For this review, take the finished solid that the model builds, in its own axes (mm). Face numbers are marked on the shaded views. A direction names the side the tool comes from. Coordinates: 2 decimals unless noted, no trailing zeros. Write each loop counter-clockwise with the first axis right and the second up, starting at its lowest first coordinate (ties: lowest second). Pieces come first, ordered by that corner, then holes. Notation, with made-up numbers: (35, 44.5) - (47, 44.5) arc R27 cw to (47, 69.5) - close; hole circle Ø2 at (31.25, -24.5). An arc over 180 degrees is marked (long way). Use one line per item in the form item = value. Start each with the question number.
1) Mouldability with a two-part tool opening along X and no side actions: class the marked faces 1 and 2 as pulls with the +X half, pulls with the -X half, needs draft (parallel to the pull), parting line crosses it, or undercut.
2) We need section B-B (z = 0). Give the boundary of the cut face in (x, y) (3 decimals), plus the area to 3 significant figures.
3) Insertion check: P1, Ø3.5, axis at x = 43.18, z = 0, coming from the +Y side; P2, Ø1.5, axis at y = 2, z = -2, coming from the +X side; P3, Ø1.5, axis at x = 40.5, y = 0.5, coming from the +Z side; P4, Ø1.6, axis at x = 29.5, y = 2, coming from the -Z side (3 decimals). Each pin has a flat end and moves straight along its axis. Give the tip position at first contact, or say it passes through.
4) We need section C-C (y = 2.7). Give the boundary of the cut face in (x, z) (3 decimals).
5) We need section D-D (x = 31.5). Give the boundary of the cut face in (y, z) (3 decimals).
6) We need section A-A (x = 43.18). Give the boundary of the cut face in (y, z) (3 decimals).
7) For L1, parallel to X at y = 1.65, z = 0 (3 decimals); L2, parallel to Z at x = 0, y = 1.05 (3 decimals); L3, parallel to X at y = 1.1, z = 1.75, list the stretches that pass through material, from the lowest coordinate up. Write a range as from..to.
8) Tool access review of the marked faces 3, 4 and 5: name each direction out of +Z, -Z, +X, -X, +Y, -Y from which nothing blocks a thin tool from reaching the whole face with its end or side.
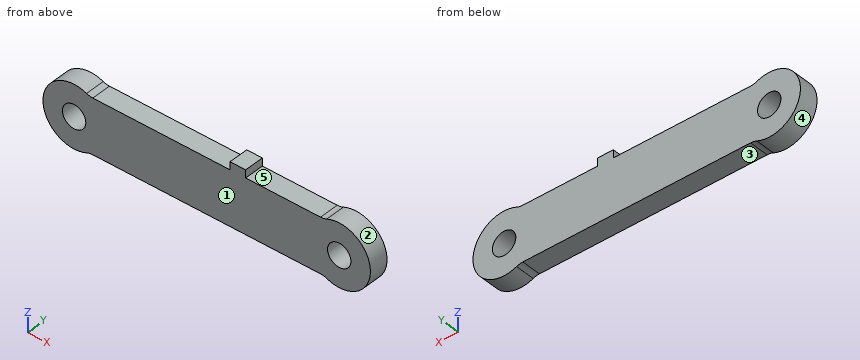
```python
from build123d import *

# Parameters (mm, degrees)
SKETCH1_R           = 5.08
SKETCH1_R_2         = 1.905
BOSS_EXTRUDE1_DEPTH = 3.175
FILLET1_R           = 2.54
SKETCH2_W           = 2.54
SKETCH2_H           = 3.175
BOSS_EXTRUDE2_DEPTH = 1.27


with BuildPart() as part:
    # Sketch1 → Boss-Extrude1 (new body)
    with BuildSketch(Plane(origin=(0, 0, 0), x_dir=(1, 0, 0), z_dir=(0, 1, 0))):
        Circle(SKETCH1_R)
        Circle(SKETCH1_R_2, mode=Mode.SUBTRACT)
        with BuildLine():
            Line((40.720655575, 4.445), (2.459344425, 4.445))
            ThreePointArc((2.459344425, 4.445), (4.376063852, 2.580012628), (5.08, 0))
            ThreePointArc((5.08, 0), (4.376063852, -2.580012628), (2.459344425, -4.445))
            Line((2.459344425, -4.445), (40.720655575, -4.445))
            ThreePointArc((40.720655575, -4.445), (38.1, 0), (40.720655575, 4.445))
        make_face()
        with Locations((43.18, 0)):
            Circle(SKETCH1_R)
        with Locations((43.18, 0)):
            Circle(SKETCH1_R_2, mode=Mode.SUBTRACT)
    extrude(amount=BOSS_EXTRUDE1_DEPTH)

    # Fillet1
    fillet1_edges = [part.edges().sort_by_distance(p)[0] for p in [
        (2.459344425, 1.5875, -4.445),
        (40.720655575, 1.5875, -4.445),
        (40.720655575, 1.5875, 4.445),
        (2.459344425, 1.5875, 4.445),
    ]]
    fillet(fillet1_edges, radius=FILLET1_R)

    # Sketch2 → Boss-Extrude2 (add)
    with BuildSketch(Plane.XY.offset(4.445)):
        with Locations((26.67, 1.5875)):
            Rectangle(SKETCH2_W, SKETCH2_H)
    extrude(amount=BOSS_EXTRUDE2_DEPTH)


solid = part.part
```
Determined:
q1.face_1 = needs draft
q1.face_2 = undercut
q2.outline = (-5.08, 0) - (-1.905, 0) - (-1.905, 3.175) - (-5.08, 3.175) - close; (1.905, 0) - (41.275, 0) - (41.275, 3.175) - (1.905, 3.175) - close; (45.085, 0) - (48.26, 0) - (48.26, 3.175) - (45.085, 3.175) - close
q2.area = 145 mm²
q3.P1 = through
q3.P2 = 48.1
q3.P3 = 4.7
q3.P4 = -4.445
q4.outline = (2.03, -4.657) arc R2.54 cw to (3.045, -4.445) - (40.135, -4.445) arc R2.54 cw to (41.15, -4.657) arc R5.08 ccw (long way) to (41.15, 4.657) arc R2.54 cw to (40.135, 4.445) - (27.94, 4.445) - (27.94, 5.715) - (25.4, 5.715) - (25.4, 4.445) - (3.045, 4.445) arc R2.54 cw to (2.03, 4.657) arc R5.08 ccw (long way) to start; hole circle Ø3.81 at (0, 0); hole circle Ø3.81 at (43.18, 0)
q5.outline = (0, -4.445) - (3.175, -4.445) - (3.175, 4.445) - (0, 4.445) - close
q6.outline = (0, -5.08) - (3.175, -5.08) - (3.175, -1.905) - (0, -1.905) - close; (0, 1.905) - (3.175, 1.905) - (3.175, 5.08) - (0, 5.08) - close
q7.L1 = -5.08..-1.905, 1.905..41.275, 45.085..48.26
q7.L2 = -5.08..-1.905, 1.905..5.08
q7.L3 = -4.77..-0.75, 0.75..42.43, 43.93..47.95
q8.face_3 = -Z, +Y, -Y
q8.face_4 = +Y, -Y
q8.face_5 = +Z, +Y, -Y
